Model file for the job. Use its own axes, mm. A direction names the side the tool comes from. Give positions to 0.01 mm unless a question says otherwise; leave off trailing zeros. Loops run counter-clockwise (first coordinate to the right, second up) from the corner with the lowest first, then second, coordinate; pieces in that order, holes last. Notation, with made-up numbers: M 40.25,11.25 L 59.25,11.25 A30 ccw 59.25,49.25 Z; hole C 88.5,85 d7. An arc over 180 degrees is marked long. Answer in a Markdown table with one row per item.
```python
from build123d import *

# Parameters (mm, degrees)
F0_R      = 76.2
F1_DEPTH  = 25.4
F2_R      = 19.05
F3_DEPTH  = 12.7
F4_R      = 5.08
F5_R      = 5.08
F6_R      = 5.715
F7_DEPTH  = 38.1
F8_R      = 5.08
F9_R      = 5.715
F10_DEPTH = 6.35
F11_R     = 7.4420743401
F13_R     = 6.3925523525
F14_DEPTH = 6.35


with BuildPart() as f1:
    # F0 (on Front) → F1 (new body)
    with BuildSketch(Plane.XZ):
        Circle(F0_R)
    extrude(amount=F1_DEPTH)

    # F2 (on face) → F3 (join)
    with BuildSketch(Plane.XZ.offset(25.4)):
        Circle(F2_R)
    extrude(amount=F3_DEPTH)

    # F4
    f4_edges = [f1.edges().sort_by_distance(p)[0] for p in [
        (-76.2, -25.4, 0),
    ]]
    fillet(f4_edges, radius=F4_R)

    # F5
    f5_edges = [f1.edges().sort_by_distance(p)[0] for p in [
        (-76.2, 0, 0),
    ]]
    fillet(f5_edges, radius=F5_R)

    # F6 (on face) → F7 (cut)
    with BuildSketch(Plane.XZ):
        Circle(F6_R)
    extrude(amount=F7_DEPTH, mode=Mode.SUBTRACT)

    # F8
    f8_edges = [f1.edges().sort_by_distance(p)[0] for p in [
        (-19.05, -38.1, 0),
    ]]
    fillet(f8_edges, radius=F8_R)

    # F9 (on face) → F10 (cut)
    with BuildSketch(Plane.XZ.offset(38.1)):
        Polygon((10.6221288443, -6.1326889476), (10.6221288443, 6.1326889476), (0, 12.2653778952), (-10.6221288443, 6.1326889476), (-10.6221288443, -6.1326889476), (0, -12.2653778952), align=None)
        Circle(F9_R, mode=Mode.SUBTRACT)
    extrude(amount=-F10_DEPTH, mode=Mode.SUBTRACT)

    # F11 (on Right) → F12 (revolve, cut)
    with BuildSketch(Plane.YZ):
        with Locations((-12.6859535106, 76.4204957727)):
            Circle(F11_R)
    revolve(axis=Axis((0, 0, 0), (0, -1, 0)), mode=Mode.SUBTRACT)

    # F13 (on face) → F14 (join)
    with BuildSketch(Plane.XZ.offset(25.4)):
        with Locations((0, 62.8129541874)):
            Circle(F13_R)
        with Locations((-44.4154658523, 44.4154658523)):
            Circle(F13_R)
        with Locations((-62.8129541874, 0)):
            Circle(F13_R)
        with Locations((-44.4154658523, -44.4154658523)):
            Circle(F13_R)
        with Locations((0, -62.8129541874)):
            Circle(F13_R)
        with Locations((44.4154658523, -44.4154658523)):
            Circle(F13_R)
        with Locations((62.8129541874, 0)):
            Circle(F13_R)
        with Locations((44.4154658523, 44.4154658523)):
            Circle(F13_R)
    extrude(amount=F14_DEPTH)


solid = f1.part
```
(1) Saw through at B-B, the plane y = -29. Count the separate pieces of the cut face and the enclosed holes in it, and give its area (3 significant figures).
Established:
| item | result |
|---|---|
| separate pieces | 9 |
| enclosed holes | 1 |
| area | 2,060 mm2 |
(2) Flat gauge pins, fed straight in: P1, Ø4, axis at y = -9.5, z = -11.5, coming from the -X side; P2, Ø7, axis at y = -36, z = 2.5, coming from the +X side; P3, Ø6.5, axis at x = 45.5, z = 47, coming from the -Y side. Where does each tip first touch, or does it go through?
Established:
| item | result |
|---|---|
| P1 | stops at x = -70.17 |
| P2 | stops at x = 19.04 |
| P3 | stops at y = -31.75 |
(3) Saw through at C-C, the plane y = -7.5. Give the cut face in (x, z) (3 decimals), and give its area (3 significant figures).
Established:
| item | result |
|---|---|
| outline | C 0,0 d142.166; hole C 0,0 d11.43 |
| area | 15,800 mm2 |
(4) Which spindle directions (+Z, -Z, +X, -X, +Y, -Y) get a long thin tool onto all of the face, cutting with end or side? Do faces 4 (the flat face through (0, -31.75, -63)), 5 (the cylindrical face through (39.343, -28.531, -48.305)), 6 (the flat face through (-63, -31.75, 0)), 7 (the flat face through (44, -31.75, 45)). Say none if no direction does.
Established:
| item | result |
|---|---|
| face 4 | -Z, +X, -X, -Y |
| face 5 | -Y |
| face 6 | +Z, -Z, -X, -Y |
| face 7 | +Z, -Z, +X, -X, -Y |
(5) Wall check: L1, parallel to Y at x = 14, z = 50.5; L2, parallel to Y at x = -43, z = 62.5; L3, parallel to X at y = -22.5, z = 2.5. Give the ranges that are in metal, low to high.
Established:
| item | result |
|---|---|
| L1 | y = -25.4 to 0 |
| L2 | y = -22.14 to -20.11, -5.26 to -3.26 |
| L3 | x = -75.67 to -5.14, 5.14 to 75.67 |
(6) Mould opens along Z. For faces 1 (the flat face through (63, -31.75, 0)), 2 (the flat face through (5.385, -34.969, 9.156)), 3 (the flat face through (-5.385, -34.969, -9.156)) say: pulls with the +Z half, pulls with the -Z half, needs draft (parallel to the pull), parting line crosses it, or undercut.
Established:
| item | result |
|---|---|
| face 1 | needs draft |
| face 2 | undercut |
| face 3 | undercut |
